Could you check a few things on this model? Use its own coordinates, in mm. Face numbers are marked on the shaded views. A direction names the side the tool comes from. Round coordinates to 2 decimals unless told otherwise and drop trailing zeros. Loops run counter-clockwise (first coordinate to the right, second up) from the corner with the lowest first, then second, coordinate; pieces in that order, holes last. Notation, with made-up numbers: M 0.5,8.5 L 31.5,8.5 A12 cw 31.5,16.5 Z; hole C 33,-7.75 d4. An arc over 180 degrees is marked long. One line per item, written item: value. Start each with the question number.
Q1. Imagine slicing it at A-A (x = 77). Please give me the cut outline in (y, z).
Q2. Imagine slicing it at B-B (y = 60.5). Please give me the cut outline in (x, z).
Q3. I'm going to push flat-ended pins straight in: pin 1 Ø8 at (x, z) = (-6.5, 15.5) entering from +Y; pin 2 Ø5 at (x, z) = (48, 4) entering from -Y; pin 3 Ø1.6 at (y, z) = (94.5, 16.5) entering from -X. Where does each tip first touch, or does it pass through?
Q4. Imagine slicing it at D-D (x = 31). Please give me the cut outline in (y, z).
Q5. Imagine slicing it at C-C (z = 8.25). Please give me the cut outline in (x, y), then the cut area to 3 significant figures.
Q6. Please list where these lines run through material, in increasing order: line 1 along Z through (x, y) = (113.5, 1.6); line 2 along X through (y, z) = (72, 6.75); line 3 along Y through (x, z) = (36, 9.75).
Q7. Thinking about a two-plate mould opening in X: for the marked faces 3, 4 and 5, which applies, released by +X, released by -X, zero draft, split by the parting line, or undercut?
Q8. Which directions (+Z, -Z, +X, -X, +Y, -Y) give clear straight access to the entire face, cutting with the end or side of a thin tool? Please do the marked faces 1 and 2.
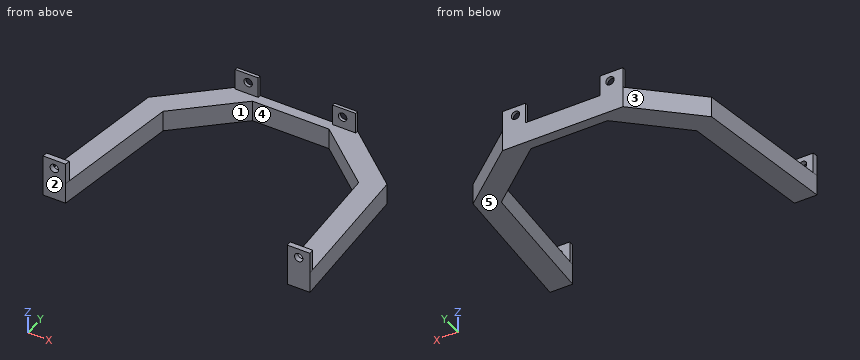
from build123d import *

# Parameters (mm, degrees)
BOSS_EXTRUDE1_DEPTH = 10
BOSS_EXTRUDE2_DEPTH = 10
SKETCH3_R           = 2.05
CUT_EXTRUDE1_DEPTH  = 10
SKETCH4_W           = 11.229416436
SKETCH4_H           = 1.5
BOSS_EXTRUDE3_DEPTH = 10
SKETCH6_R           = 2.05
CUT_EXTRUDE2_DEPTH  = 10


with BuildPart() as part:
    # Sketch1 → Boss-Extrude1 (new body)
    with BuildSketch(Plane.XY):
        Polygon((0, 0), (-11, 0), (-2.811023481, 69.662685047), (24.646347311, 95), (83.353652689, 95), (113.374131029, 69.662685047), (119, 0), (108, 0), (102.791775395, 64.491176779), (72.568088456, 90), (35.224285945, 90), (7.581056228, 64.491176779), align=None)
    extrude(amount=BOSS_EXTRUDE1_DEPTH)

    # Sketch2 → Boss-Extrude2 (add)
    with BuildSketch(Plane.XY.offset(10)):
        Polygon((-11, 0), (0, 0), (0.29387959, 2.5), (-10.70612041, 2.5), align=None)
        Polygon((108, 0), (119, 0), (118.798103211, 2.5), (107.798103211, 2.5), align=None)
    extrude(amount=BOSS_EXTRUDE2_DEPTH)

    # Sketch3 → Cut-Extrude1 (cut)
    with BuildSketch(Plane(origin=(0, 2.5, 0), x_dir=(1, 0, 0), z_dir=(0, 1, 0))):
        with Locations(Location((-5.5, -15.687372709, 0), (0, 0, 180))):
            Circle(SKETCH3_R)
        with Locations(Location((113.5, -15.687372709, 0), (0, 0, 180))):
            Circle(SKETCH3_R)
    extrude(amount=-CUT_EXTRUDE1_DEPTH, mode=Mode.SUBTRACT)

    # Sketch4 → Boss-Extrude3 (add)
    with BuildSketch(Plane.XY.offset(10)):
        with Locations((30.261055529, 94.25)):
            Rectangle(SKETCH4_W, SKETCH4_H)
        with Locations((77.738944471, 94.25)):
            Rectangle(SKETCH4_W, SKETCH4_H)
    extrude(amount=BOSS_EXTRUDE3_DEPTH)

    # Sketch6 → Cut-Extrude2 (cut)
    with BuildSketch(Plane(origin=(0, 95, 0), x_dir=(1, 0, 0), z_dir=(0, 1, 0))):
        with Locations(Location((31, -15.687372709, 0), (0, 0, 270))):
            Circle(SKETCH6_R)
        with Locations(Location((77, -15.687372709, 0), (0, 0, 270))):
            Circle(SKETCH6_R)
    extrude(amount=-CUT_EXTRUDE2_DEPTH, mode=Mode.SUBTRACT)


solid = part.part
Report:
1. outline: M 86.26,0 L 95,0 L 95,13.64 L 93.5,13.64 L 93.5,10 L 86.26,10 Z; M 93.5,17.74 L 95,17.74 L 95,20 L 93.5,20 Z
2. outline: M -3.89,0 L 7.11,0 L 7.11,10 L -3.89,10 Z; M 103.11,0 L 114.11,0 L 114.11,10 L 103.11,10 Z
3. pin 1: stops at y = 2.5
3. pin 2: stops at y = 90
3. pin 3: stops at x = 24.65
4. outline: M 86.1,0 L 95,0 L 95,13.64 L 93.5,13.64 L 93.5,10 L 86.1,10 Z; M 93.5,17.74 L 95,17.74 L 95,20 L 93.5,20 Z
5. outline: M -11,0 L 0,0 L 7.58,64.49 L 35.22,90 L 72.57,90 L 102.79,64.49 L 108,0 L 119,0 L 113.37,69.66 L 83.35,95 L 24.65,95 L -2.81,69.66 Z
5. area: 2,550 mm²
6. line 1: z = 0 to 13.64, 17.74 to 20
6. line 2: x = -0.28 to 15.72, 93.9 to 110.6
6. line 3: y = 90 to 95
7. face 3: released by -X
7. face 4: undercut
7. face 5: zero draft
8. face 1: +Z, -Z, -Y
8. face 2: +Z, -Z, +X, -X, -Y
